Check sheet for the drawn part. Datum: minimum x, y, z corner. Units: mm. Round coordinates to 2 decimals unless told otherwise and drop trailing zeros. Write each loop counter-clockwise with the first axis right and the second up, starting at its lowest first coordinate (ties: lowest second). Pieces come first, ordered by that corner, then holes. Notation, with made-up numbers: M 35,67.25 L 91,67.25 A34 ccw 91,98.25 Z; hole C 7,41.25 d11. An arc over 180 degrees is marked long. One line per item, written item: value. Start each with the question number.
Item 1: Gauge pin test, flat end, axial feed: pin 1 (3.5 mm diameter, centred on x = 4, z = 52, fed in from +Y). Record the tip position at first contact, or that the pin passes through.
Item 2: Section check A-A, the plane x = 44. State how many separate pieces and enclosed holes the cut face has, then the cut area to 3 significant figures.
Item 3: Thickness scan on probe 1 along X at (y, z) = (0.75, 46.5); probe 2 along Z at (x, y) = (24.5, 1.1); probe 3 along X at (y, z) = (2.2, 25.5). Record the ranges inside material, lowest first. Write a range as from..to.
Item 4: Section check B-B, the plane z = 15. Record the cut outline in (x, y), then the cut area to 3 significant figures.
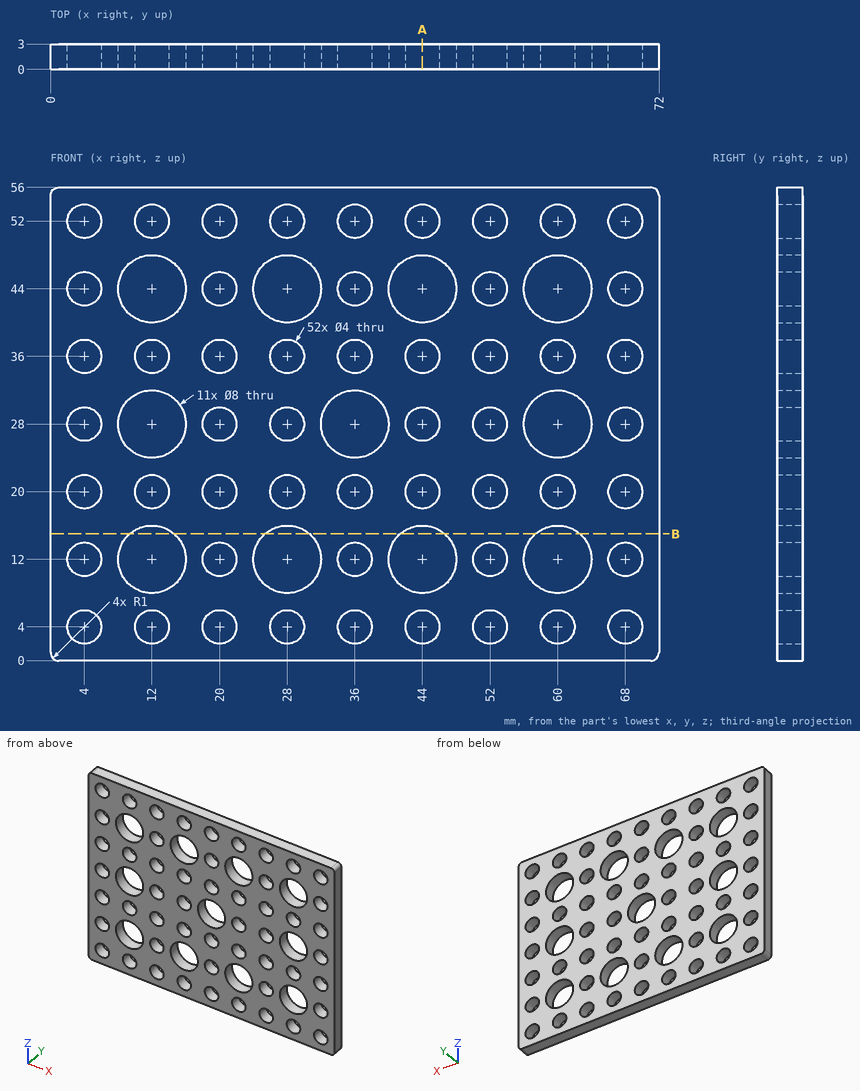
Response values:
1. pin 1: passes through
2. separate pieces: 8
2. enclosed holes: 0
2. area: 60.0 mm2
3. probe 1: x = 0..8.88, 15.12..24.88, 31.12..40.88, 47.12..56.88, 63.12..72
3. probe 2: z = 0..10.06, 13.94..42.06, 45.94..56
3. probe 3: x = 0..8.88, 15.12..32.88, 39.12..56.88, 63.12..72
4. outline: M 0,0 L 9.35,0 L 9.35,3 L 0,3 Z; M 14.65,0 L 25.35,0 L 25.35,3 L 14.65,3 Z; M 30.65,0 L 41.35,0 L 41.35,3 L 30.65,3 Z; M 46.65,0 L 57.35,0 L 57.35,3 L 46.65,3 Z; M 62.65,0 L 72,0 L 72,3 L 62.65,3 Z
4. area: 153 mm2
